from build123d import *

# Parameters (mm, degrees)
SKETCH1_R           = 2.032
BOSS_EXTRUDE1_DEPTH = 3.175
SKETCH1_3_R         = 2.032
CUT_EXTRUDE2_DEPTH  = 270.126904313
FILLET1_R           = 3.81
FILLET2_R           = 10.16
FILLET3_R           = 12.7
FILLET4_R           = 1.27
FILLET5_R           = 2.54
FILLET6_DEPTH       = 3.175


with BuildPart() as part:
    # Sketch1 → Boss-Extrude1 (new body)
    with BuildSketch(Plane(origin=(0, 0, 0), x_dir=(1, 0, 0), z_dir=(0, 1, 0))):
        Polygon((0, 0), (254, 0), (254, 12.7), (203.2, 88.9), (152.4, 88.9), (0, 12.7), align=None)
        with Locations(Location((12.7, 6.35, 0), (0, 0, 270))):
            Circle(SKETCH1_R, mode=Mode.SUBTRACT)
        with Locations(Location((25.4, 6.35, 0), (0, 0, 270))):
            Circle(SKETCH1_R, mode=Mode.SUBTRACT)
        with Locations(Location((228.6, 6.35, 0), (0, 0, 270))):
            Circle(SKETCH1_R, mode=Mode.SUBTRACT)
        with Locations(Location((241.3, 6.35, 0), (0, 0, 270))):
            Circle(SKETCH1_R, mode=Mode.SUBTRACT)
        with Locations(Location((162.983333333, 82.55, 0), (0, 0, 270))):
            Circle(SKETCH1_R, mode=Mode.SUBTRACT)
        with Locations(Location((188.383333333, 82.55, 0), (0, 0, 270))):
            Circle(SKETCH1_R, mode=Mode.SUBTRACT)
    extrude(amount=BOSS_EXTRUDE1_DEPTH)

    # Sketch1<3> → Cut-Extrude2 (cut, through all)
    with BuildSketch(Plane(origin=(0, 0, 0), x_dir=(1, 0, 0), z_dir=(0, 1, 0))):
        Polygon((115.724624488, 64.882699581), (27.28853263, 20.664653652), (35.82613579, 14.323081227), align=None)
        Polygon((197.627677458, 6.91131175), (198.543333333, 5.08), (216.209513725, 5.08), (196.001097378, 33.83556314), align=None)
        with Locations(Location((162.983333333, 6.35, 0), (0, 0, 270))):
            Circle(SKETCH1_3_R)
        Polygon((190.635905135, 38.402947882), (156.633333333, 12.7), (192.188702367, 12.7), align=None)
        Polygon((94.175435772, 32.591444541), (43.396541726, 5.08), (94.175435772, 5.08), align=None)
        with Locations(Location((188.383333333, 6.35, 0), (0, 0, 270))):
            Circle(SKETCH1_3_R)
        Polygon((99.255435772, 30.509658634), (99.255435772, 5.08), (123.491206376, 5.08), align=None)
        Polygon((163.49857777, 76.2), (140.931419259, 76.2), (139.042658246, 64.374485547), align=None)
        Polygon((191.431375489, 49.173139927), (220.831581656, 7.338120783), (225.073834238, 13.650530069), align=None)
        Polygon((182.993969781, 52.344053487), (145.913976972, 18.776250855), (189.241078693, 43.454730757), align=None)
        Polygon((134.963762863, 71.045523698), (77.053379688, 34.399938534), (133.467710225, 61.678752584), align=None)
        Polygon((229.214596962, 15.811166321), (245.82048896, 15.811166321), (211.171400328, 67.784799269), align=None)
        Polygon((132.104025549, 53.140736008), (100.845083482, 36.204986082), (125.300627654, 10.544727526), align=None)
        Polygon((169.510067662, 71.530970072), (137.832506287, 18.312666963), (180.050783748, 56.53205963), align=None)
        Polygon((186.192725225, 62.092240839), (201.77657544, 76.2), (172.831665677, 76.2), align=None)
        Polygon((162.432346465, 69.572285661), (137.735749394, 56.191941851), (131.599534907, 17.773162244), align=None)
        Polygon((189.686775345, 58.402921334), (220.256823492, 26.124427609), (204.420515632, 71.741092366), align=None)
    extrude(amount=CUT_EXTRUDE2_DEPTH, mode=Mode.SUBTRACT)

    # Fillet1
    fillet1_edges = [part.edges().sort_by_distance(p)[0] for p in [
        (0, 1.5875, 0),
        (254, 1.5875, 0),
    ]]
    fillet(fillet1_edges, radius=FILLET1_R)

    # Fillet2
    fillet2_edges = [part.edges().sort_by_distance(p)[0] for p in [
        (254, 1.5875, -12.7),
        (0, 1.5875, -12.7),
    ]]
    fillet(fillet2_edges, radius=FILLET2_R)

    # Fillet3
    fillet3_edges = [part.edges().sort_by_distance(p)[0] for p in [
        (203.2, 1.5875, -88.9),
        (152.4, 1.5875, -88.9),
    ]]
    fillet(fillet3_edges, radius=FILLET3_R)

    # Fillet4
    fillet4_edges = [part.edges().sort_by_distance(p)[0] for p in [
        (220.256823492, 1.5875, -26.124427609),
        (211.171400328, 1.5875, -67.784799269),
        (191.431375489, 1.5875, -49.173139927),
        (115.724624488, 1.5875, -64.882699581),
        (77.053379688, 1.5875, -34.399938534),
    ]]
    fillet(fillet4_edges, radius=FILLET4_R)

    # Fillet5
    fillet5_edges = [part.edges().sort_by_distance(p)[0] for p in [
        (172.831665677, 1.5875, -76.2),
        (204.420515632, 1.5875, -71.741092366),
        (131.599534907, 1.5875, -17.773162244),
        (162.432346465, 1.5875, -69.572285661),
        (137.735749394, 1.5875, -56.191941851),
        (169.510067662, 1.5875, -71.530970072),
        (137.832506287, 1.5875, -18.312666963),
        (196.001097378, 1.5875, -33.83556314),
        (198.543333333, 1.5875, -5.08),
        (216.209513725, 1.5875, -5.08),
        (145.913976972, 1.5875, -18.776250855),
        (189.241078693, 1.5875, -43.454730757),
        (245.82048896, 1.5875, -15.811166321),
        (220.831581656, 1.5875, -7.338120783),
        (94.175435772, 1.5875, -32.591444541),
        (43.396541726, 1.5875, -5.08),
        (27.28853263, 1.5875, -20.664653652),
        (140.931419259, 1.5875, -76.2),
        (139.042658246, 1.5875, -64.374485547),
        (163.49857777, 1.5875, -76.2),
        (134.963762863, 1.5875, -71.045523698),
        (133.467710225, 1.5875, -61.678752584),
        (123.491206376, 1.5875, -5.08),
        (99.255435772, 1.5875, -30.509658634),
        (125.300627654, 1.5875, -10.544727526),
        (132.104025549, 1.5875, -53.140736008),
        (100.845083482, 1.5875, -36.204986082),
        (190.635905135, 1.5875, -38.402947882),
        (156.633333333, 1.5875, -12.7),
        (192.188702367, 1.5875, -12.7),
        (201.77657544, 1.5875, -76.2),
    ]]
    fillet(fillet5_edges, radius=FILLET5_R)

    # Fillet6: read off the stored shape, not the designer's step
    # Fillet6 outline → Fillet6 (add)
    with BuildSketch(Plane(origin=(0, 0, 0), x_dir=(1, 0, 0), z_dir=(0, 1, 0))):
        with BuildLine():
            Line((197.627677458, 6.91131175), (197.8412946, 6.484077467))
            ThreePointArc((197.8412946, 6.484077467), (197.660329187, 7.15163193), (197.571718595, 7.837580619))
            Line((197.571718595, 7.837580619), (197.627677458, 6.91131175))
        make_face()
        with BuildLine():
            ThreePointArc((38.77257119, 16.18758019), (35.866508895, 15.403840031), (33.027019658, 16.402212494))
            Line((33.027019658, 16.402212494), (35.82613579, 14.323081227))
            Line((35.82613579, 14.323081227), (38.77257119, 16.18758019))
        make_face()
        with BuildLine():
            Line((229.214596962, 15.811166321), (232.828436892, 15.811166321))
            ThreePointArc((232.828436892, 15.811166321), (229.883700891, 16.751730382), (228.029403022, 19.225130932))
            Line((228.029403022, 19.225130932), (229.214596962, 15.811166321))
        make_face()
        with BuildLine():
            Line((225.073834238, 13.650530069), (222.279686918, 16.600831826))
            ThreePointArc((222.279686918, 16.600831826), (223.646593023, 13.608087476), (222.892967422, 10.405432406))
            Line((222.892967422, 10.405432406), (225.073834238, 13.650530069))
        make_face()
        with BuildLine():
            Line((94.175435772, 5.08), (94.175435772, 10.16))
            ThreePointArc((94.175435772, 10.16), (92.687538221, 6.567897552), (89.095435772, 5.08))
            Line((89.095435772, 5.08), (94.175435772, 5.08))
        make_face()
        with BuildLine():
            ThreePointArc((104.335435772, 5.08), (100.743333324, 6.567897552), (99.255435772, 10.16))
            Line((99.255435772, 10.16), (99.255435772, 5.08))
            Line((99.255435772, 5.08), (104.335435772, 5.08))
        make_face()
        with BuildLine():
            Line((189.686775345, 58.402921334), (193.259422183, 54.630612636))
            ThreePointArc((193.259422183, 54.630612636), (191.871557973, 58.31892969), (193.538494235, 61.889808188))
            Line((193.538494235, 61.889808188), (189.686775345, 58.402921334))
        make_face()
        with BuildLine():
            ThreePointArc((189.874971747, 65.425707626), (186.270506771, 64.115486966), (182.777271822, 65.69857115))
            Line((182.777271822, 65.69857115), (186.192725225, 62.092240839))
            Line((186.192725225, 62.092240839), (189.874971747, 65.425707626))
        make_face()
        with BuildLine():
            Line((180.050783748, 56.53205963), (177.469122224, 60.205634526))
            ThreePointArc((177.469122224, 60.205634526), (178.361429352, 56.720772492), (176.722145031, 53.518707171))
            Line((176.722145031, 53.518707171), (180.050783748, 56.53205963))
        make_face()
        with BuildLine():
            ThreePointArc((178.733075257, 48.486747819), (182.706353411, 49.769316538), (186.298680322, 47.641616097))
            Line((186.298680322, 47.641616097), (182.993969781, 52.344053487))
            Line((182.993969781, 52.344053487), (178.733075257, 48.486747819))
        make_face()
    extrude(amount=FILLET6_DEPTH)


solid = part.part
Geometry: final body of the model. Coordinates: model frame, mm. A direction names the side the tool comes from. Round coordinates to 2 decimals unless told otherwise and drop trailing zeros. Order: outer loops, then holes, each group sorted by start corner. A loop starts at its lowest first (then second) coordinate and runs counter-clockwise, first axis right, second up. Notation, with made-up numbers: (39.5, -26) -> (92.5, -26) arc R13 ccw to (92.5, -5) -> close; hole circle Ø11 at (1.25, -39.5). An arc over 180 degrees is marked (long way). Put each result on its own line as item: value. Start each with the question number.
Q1. First-contact query: pin 1 (3.5 mm diameter, centred on x = 162.98, z = -6.35, fed in from -Y); pin 2 (1 mm diameter, centred on x = 235, y = 1.5, fed in from -Z); pin 3 (1 mm diameter, centred on y = 1.5, z = -22, fed in from -X); pin 4 (1 mm diameter, centred on y = 1.5, z = -14, fed in from +X). Flat tips, straight axial feed; report the tip coordinate or a pass-through.
Q2. Section C-C on y = 1.8. Give the number of separate pieces and of enclosed holes in the cut face, and give its area (3 significant figures).
Q3. Reachability of faces 5 (the flat face through (163.36, 1.57, -41.42)), 6 (the flat face through (229.949, 1.565, -48.776)) from +Z, -Z, +X, -X, +Y, -Y: full face, straight path, thin tool, end or side. Return the list, or none.
Q4. Pull-direction query (X, two-part tool) for faces 1 (the flat face through (176.304, 1.565, -36.086)), 2 (the cylindrical face through (1.48, 1.61, -11.7)), 3 (the flat face through (111.628, 1.565, -17.528)), 4 (the flat face through (153, 3.175, -45)); classes: +X half, -X half, draft (parallel to the pull), parting line (faces both ways), or undercut.
Q5. Section A-A on x = 69. Return the cut outline in (y, z) (3 decimals).
Q6. Line query: probe 1 along Z at (x, y) = (70, 1.1); probe 2 along Z at (x, y) = (84, 1.3); probe 3 along X at (y, z) = (1.45, -82). Output: solid intervals per line, ascending.
Q7. Section B-B on x = 111. Return the cut outline in (y, z) (3 decimals), and give its area (3 significant figures).
Ans:
1. pin 1: passes through
1. pin 2: stops at z = -41.95
1. pin 3: stops at x = 17.6
1. pin 4: stops at x = 253.23
2. separate pieces: 1
2. enclosed holes: 23
2. area: 9,470 mm2
3. face 5: +Y, -Y
3. face 6: -Z, +X, +Y, -Y
4. face 1: undercut
4. face 2: -X half
4. face 3: undercut
4. face 4: draft
5. outline: (0, -47.2) -> (3.175, -47.2) -> (3.175, -41.52) -> (0, -41.52) -> close; (0, -35.315) -> (3.175, -35.315) -> (3.175, -18.952) -> (0, -18.952) -> close; (0, -5.08) -> (3.175, -5.08) -> (3.175, 0) -> (0, 0) -> close
6. probe 1: z = -47.7 to -42.02, -35.95 to -19.49, -5.08 to 0
6. probe 2: z = -54.7 to -49.02, -44.81 to -27.08, -5.08 to 0
6. probe 3: x = 138.6 to 161.03, 164.94 to 186.43, 190.34 to 207.8
7. outline: (0, -68.2) -> (3.175, -68.2) -> (3.175, -55.881) -> (0, -55.881) -> close; (0, -50.815) -> (3.175, -50.815) -> (3.175, -41.707) -> (0, -41.707) -> close; (0, -25.55) -> (3.175, -25.55) -> (3.175, -18.187) -> (0, -18.187) -> close; (0, -5.08) -> (3.175, -5.08) -> (3.175, 0) -> (0, 0) -> close
7. area: 108 mm2
